Input: part model. Units: mm. Frame: model coordinates. Give positions to 0.01 mm unless a question says otherwise; leave off trailing zeros. Loops run counter-clockwise (first coordinate to the right, second up) from the corner with the lowest first, then second, coordinate; pieces in that order, holes last.
from build123d import *

# Parameters (mm, degrees)
F0_W     = 120
F0_H     = 40
F1_DEPTH = 3
F2_R     = 1
F3_R     = 0.75
F4_DEPTH = 5.9
F5_W     = 4.308377
F5_H     = 3.907596
F5_W_2   = 4.308376
F6_DEPTH = 4


with BuildPart() as f1:
    # F0 (on Front) → F1 (new body)
    with BuildSketch(Plane.XZ):
        Rectangle(F0_W, F0_H)
    extrude(amount=F1_DEPTH)

    # F2
    f2_edges = [f1.edges().sort_by_distance(p)[0] for p in [
        (0, -3, 20),
        (-60, -3, 0),
        (0, -3, -20),
        (60, -3, 0),
    ]]
    fillet(f2_edges, radius=F2_R)

    # F3 (on face) → F4 (cut)
    with BuildSketch(Plane.XZ.offset(3)):
        with Locations((-45, 13)):
            Circle(F3_R)
        with Locations((-29, 13)):
            Circle(F3_R)
        with Locations((28.25, 13)):
            Circle(F3_R)
        with Locations((44.25, 13)):
            Circle(F3_R)
    extrude(amount=-F4_DEPTH, mode=Mode.SUBTRACT)

    # F5 (on face) → F6 (join)
    with BuildSketch(Plane(origin=(0, 0, 0), x_dir=(-1, 0, 0), z_dir=(0, 1, 0))):
        with Locations((-44.288592, 12.487537)):
            Rectangle(F5_W, F5_H)
        with Locations((-28.407722, 12.487537)):
            Rectangle(F5_W, F5_H)
        with Locations((28.944263, 12.487537)):
            Rectangle(F5_W_2, F5_H)
        with Locations((45.069936, 12.487537)):
            Rectangle(F5_W, F5_H)
    extrude(amount=F6_DEPTH)


solid = f1.part
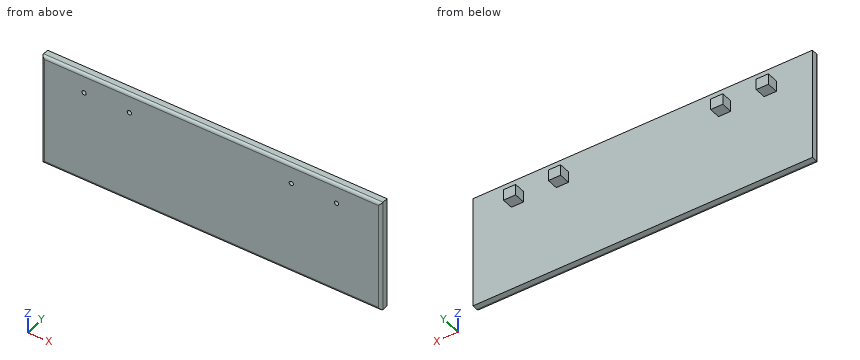
(1) Ray query, probe 1 along X at (y, z) = (3.5, 11); probe 2 along Z at (x, y) = (-45, -2.2); probe 3 along Y at (x, z) = (52, -16.5). Return the intervals inside material, ascending.
Values follow:
probe 1: x = -47.22 to -42.92, -31.1 to -26.79, 26.25 to 30.56, 42.13 to 46.44
probe 2: z = -19.98 to 12.25, 13.75 to 19.98
probe 3: y = -3 to 0
(2) Cut plane A-A (y = 2). Return the cut outline in (x, z).
Values follow:
outline: (-47.22, 10.53) - (-42.92, 10.53) - (-42.92, 14.44) - (-47.22, 14.44) - close; (-31.1, 10.53) - (-26.79, 10.53) - (-26.79, 14.44) - (-31.1, 14.44) - close; (26.25, 10.53) - (30.56, 10.53) - (30.56, 14.44) - (26.25, 14.44) - close; (42.13, 10.53) - (46.44, 10.53) - (46.44, 14.44) - (42.13, 14.44) - close
(3) Cut plane B-B (z = -13.5). Return the cut outline in (x, y), and give its area (3 significant figures).
Values follow:
outline: (-60, -2) arc R1 ccw to (-59, -3) - (59, -3) arc R1 ccw to (60, -2) - (60, 0) - (-60, 0) - close
area: 360 mm2
(4) Pin query (flat end, axial travel): pin 1 Ø2 at (y, z) = (1.5, 11.5) entering from +X; pin 2 Ø2 at (y, z) = (2.5, 11.5) entering from -X; pin 3 Ø0.9 at (x, z) = (28.25, 13) entering from -Y; pin 4 Ø1 at (x, y) = (25, 3) entering from -Z. Return the tip coordinate at first contact, or that it passes through.
Values follow:
pin 1: stops at x = 46.44
pin 2: stops at x = -47.22
pin 3: stops at y = 0
pin 4: passes through
(5) Cut plane C-C (x = 12.5). Return the cut outline in (y, z), and give its area (3 significant figures).
Values follow:
outline: (-3, -19) arc R1 ccw to (-2, -20) - (0, -20) - (0, 20) - (-2, 20) arc R1 ccw to (-3, 19) - close
area: 120 mm2
